Design review of the part built by this model. Coordinates are the model's own, in mm. A direction names the side the tool comes from. Give positions to 0.01 mm unless a question says otherwise; leave off trailing zeros. Loops run counter-clockwise (first coordinate to the right, second up) from the corner with the lowest first, then second, coordinate; pieces in that order, holes last.
from build123d import *

# Parameters (mm, degrees)
F0_R     = 19.2346
F1_DEPTH = 16.764
F2_R     = 16.832332
F3_DEPTH = 20.828
F4_R     = 14.200523
F5_DEPTH = 25.4
F6_R     = 11.141094
F7_DEPTH = 39.624
F9_D     = 19.05


with BuildPart() as f1:
    # F0 (on Top) → F1 (new body)
    with BuildSketch(Plane.XY):
        Circle(F0_R)
    extrude(amount=F1_DEPTH)

    # F2 (on Top) → F3 (join)
    with BuildSketch(Plane.XY):
        Circle(F2_R)
    extrude(amount=F3_DEPTH)

    # F4 (on Top) → F5 (join)
    with BuildSketch(Plane.XY):
        Circle(F4_R)
    extrude(amount=F5_DEPTH)

    # F6 (on Top) → F7 (join)
    with BuildSketch(Plane.XY):
        Circle(F6_R)
    extrude(amount=F7_DEPTH)

    # F9 (through all)
    with Locations(Plane.XY.offset(39.624)):
        with Locations((0, 0)):
            Hole(F9_D / 2)


solid = f1.part
Q1. Take a section at D-D (x = 12.5). Give the boundary of the cut face in (y, z).
Results:
outline: (-14.62, 0) - (14.62, 0) - (14.62, 16.76) - (11.27, 16.76) - (11.27, 20.83) - (6.74, 20.83) - (6.74, 25.4) - (-6.74, 25.4) - (-6.74, 20.83) - (-11.27, 20.83) - (-11.27, 16.76) - (-14.62, 16.76) - close
Q2. Insertion check: pin 1 (5 mm diameter, centred on y = -10, z = 10.5, fed in from +X); pin 2 (12 mm diameter, centred on x = 10, z = 11, fed in from -Y); pin 3 (5 mm diameter, centred on x = -12.5, z = 23, fed in from +Y); pin 4 (8 mm diameter, centred on x = 2.5, y = -3, fed in from -Z). Each pin has a flat end and moves straight along its axis. Give the tip position at first contact, or say it passes through.
Results:
pin 1: stops at x = 17.71
pin 2: stops at y = -18.81
pin 3: stops at y = 12.51
pin 4: passes through
Q3. Draft analysis for pull direction Y (two halves, no side actions). For faces 1 (the face through (-1.85, 14.08, 23.08)), 2 (the face through (-5, 8.3, 39.624)), 3 (the face through (7.559, -5.796, 19.535)), state which applies: pulls with the +Y half, pulls with the -Y half, needs draft (parallel to the pull), parting line crosses it, or undercut.
Results:
face 1: parting line crosses it
face 2: needs draft
face 3: undercut
Q4. Take a section at C-C (z = 7). Give the boundary of the cut face in (x, y) (3 decimals), plus the area to 3 significant figures.
Results:
outline: circle Ø38.469 at (0, 0); hole circle Ø19.05 at (0, 0)
area: 877 mm2
Q5. Take a section at A-A (y = 0). Give the boundary of the cut face in (x, z) (3 decimals).
Results:
outline: (-19.235, 0) - (-9.525, 0) - (-9.525, 39.624) - (-11.141, 39.624) - (-11.141, 25.4) - (-14.201, 25.4) - (-14.201, 20.828) - (-16.832, 20.828) - (-16.832, 16.764) - (-19.235, 16.764) - close; (9.525, 0) - (19.235, 0) - (19.235, 16.764) - (16.832, 16.764) - (16.832, 20.828) - (14.201, 20.828) - (14.201, 25.4) - (11.141, 25.4) - (11.141, 39.624) - (9.525, 39.624) - close
Q6. Tool access review of faces 4 (the face through (-9, -4, 0)), 5 (the face through (-3.65, -16.43, 18.77)): name each direction out of +Z, -Z, +X, -X, +Y, -Y from which nothing blocks a thin tool from reaching the whole face with its end or side.
Results:
face 4: -Z, +X, -X, +Y, -Y
face 5: +Z
Q7. Wall thickness on line 1 (Y direction, x = 0, z = 30) (3 decimals); line 2 (Y direction, x = 0, z = 16) (3 decimals); line 3 (Z direction, x = -1, y = -11.5): over which ranges is each line inside the solid? List them lowest first.
Results:
line 1: y = -11.141 to -9.525, 9.525 to 11.141
line 2: y = -19.235 to -9.525, 9.525 to 19.235
line 3: z = 0 to 25.4
